Check sheet for the modelled part. Datum: model origin and axes. Units: mm. A direction names the side the tool comes from. Give positions to 0.01 mm unless a question says otherwise; leave off trailing zeros. Write each loop counter-clockwise with the first axis right and the second up, starting at its lowest first coordinate (ties: lowest second). Pieces come first, ordered by that corner, then holes. Notation, with made-up numbers: M -30.75,14.5 L -18.75,14.5 A6 cw -18.75,25.5 Z; hole C 88.5,-23.5 d7. An arc over 180 degrees is marked long. Write item = value, one per line. Start each with the question number.
1) Sectioned sample at B-B, the plane y = 0. Record the cut outline in (x, z).
2) Scan lines: L1, parallel to X at y = 0, z = -3.65; L2, parallel to Z at x = 4, y = 18; L3, parallel to Y at x = 4, z = -15. Record each from-to range of solid material in increasing order.
3) Sectioned sample at A-A, the plane z = 0. Record the cut outline in (x, y), then the cut area to 3 significant figures.
4) Sectioned sample at D-D, the plane y = -12.5. Record the cut outline in (x, z), then the cut area to 3 significant figures.
5) Draft check along Z on faces 1 (the face through (3.549, 21.728, -3.449)), 2 (the face through (-2, 2.48, -5.71)), 3 (the face through (3.45, 10.31, 16.93)). Enter one of: pulls with the +Z half, pulls with the -Z half, needs draft (parallel to the pull), parting line crosses it, or undercut.
6) Set-up check for faces 4 (the face through (3.45, 10.27, -14.17)), 5 (the face through (3.451, 19.816, -1.634)), 6 (the face through (3.451, 1.634, 19.816)): record each of +Z, -Z, +X, -X, +Y, -Y from which the full face is reachable in a straight line by a thin tool's end or side.
7) Gauge pin test, flat ends, axial feed: pin 1 (4 mm diameter, centred on x = 2.5, y = 0.5, fed in from -Z); pin 2 (2.5 mm diameter, centred on x = -2, y = 1.5, fed in from -Z); pin 3 (1.5 mm diameter, centred on y = 11.5, z = 1.5, fed in from -X). Record the tip position at first contact, or that the pin passes through.
8) Sectioned sample at C-C, the plane x = -2.5. Record the cut outline in (y, z).
from build123d import *

# Parameters (mm, degrees)
BASPROSKE_W              = 7
BASPROSKE_H              = 22
TOOTHCUT_DEPTH           = 32.890437438
TEETHCUTS_COUNT          = 20
TEETHCUTS_ANGLE          = 342
HUBNEAONESKE_R           = 7
HUBNEARONE_DEPTH         = 6.0000508
BORSKE_R                 = 3
BORE_DEPTH               = 13.0000508
CUT_EXTRUDE_3_DEPTH      = 34.466904857
CUT_EXTRUDE_3_DEPTH_BACK = 34.466904857
SKETCH_4_R               = 3.15
EXTRUDE_1_DEPTH          = 13.000051
CUT_EXTRUDE_4_DEPTH      = 32.623288929
CUT_EXTRUDE_4_DEPTH_BACK = 32.623288929
SKETCH_2_R               = 1.65
CUT_EXTRUDE_5_DEPTH      = 2


with BuildPart() as part:
    # BasProSke → Base-Revolve (revolve)
    with BuildSketch(Plane(origin=(0, 0, 0), x_dir=(1, 0, 0), z_dir=(0, 1, 0)), mode=Mode.PRIVATE) as base_revolve_sk:
        with Locations((3.5, 11)):
            Rectangle(BASPROSKE_W, BASPROSKE_H)
    revolve(base_revolve_sk.sketch.rotate(Axis((-10, 0, 0), (1, 0, 0)), 180), axis=Axis((-10, 0, 0), (1, 0, 0)))

    # TooCutSke → ToothCut (cut, through all)
    with BuildSketch(Plane(origin=(0, 0, 0), x_dir=(0, 0, -1), z_dir=(1, 0, 0))):
        with BuildLine():
            ThreePointArc((0.986171591, 17.471189616), (0, 17.499), (-0.986171591, 17.471189616))
            ThreePointArc((-0.986171591, 17.471189616), (-1.626916196, 19.798789858), (-2.932850173, 21.829260982))
            ThreePointArc((-2.932850173, 21.829260982), (0, 22.0254), (2.932850173, 21.829260982))
            ThreePointArc((2.932850173, 21.829260982), (1.626916196, 19.798789858), (0.986171591, 17.471189616))
        make_face()
    toothcut = extrude(amount=TOOTHCUT_DEPTH, mode=Mode.SUBTRACT)

    # TeethCuts: ToothCut ×20 about axis
    teethcuts_axis = Axis((-10, 0, 0), (1, 0, 0))
    for i in range(1, TEETHCUTS_COUNT):
        add(toothcut.rotate(teethcuts_axis, i * TEETHCUTS_ANGLE / (TEETHCUTS_COUNT - 1)), mode=Mode.SUBTRACT)

    # HubNeaOneSke → HubNearOne (add)
    with BuildSketch(Plane.ZY):
        with Locations(Location((0, 0, 0), (0, 0, 180))):
            Circle(HUBNEAONESKE_R)
    extrude(amount=HUBNEARONE_DEPTH)

    # BorSke → Bore (cut, symmetric)
    with BuildSketch(Plane(origin=(0, 0, 0), x_dir=(0, 0, -1), z_dir=(1, 0, 0))):
        with Locations(Location((0, 0, 0), (0, 0, 180))):
            Circle(BORSKE_R)
    extrude(amount=BORE_DEPTH, both=True, mode=Mode.SUBTRACT)

    # 草图4 → 切除-拉伸3 (cut, two sides: drawn at the far end of the back side and taken through both)
    with BuildSketch(Plane.ZY.offset(6.0000508).offset(-CUT_EXTRUDE_3_DEPTH_BACK)):
        Circle(SKETCH_4_R)
    extrude(amount=CUT_EXTRUDE_3_DEPTH + CUT_EXTRUDE_3_DEPTH_BACK, mode=Mode.SUBTRACT)

    # 草图1 → 凸台-拉伸1 (add, through all)
    with BuildSketch(Plane.ZY.offset(6.0000508)):
        with BuildLine():
            Line((2.6, 1.778341924), (2.6, -1.778341924))
            ThreePointArc((2.6, -1.778341924), (3.15, 0), (2.6, 1.778341924))
        make_face()
    extrude(amount=-EXTRUDE_1_DEPTH)

    # 草图2 → 切除-拉伸4 (cut, two sides: drawn at the far end of the back side and taken through both)
    with BuildSketch(Plane.XY.offset(-CUT_EXTRUDE_4_DEPTH_BACK)):
        with Locations((-3.5000508, 0)):
            Circle(SKETCH_2_R)
    extrude(amount=CUT_EXTRUDE_4_DEPTH + CUT_EXTRUDE_4_DEPTH_BACK, mode=Mode.SUBTRACT)

    # 草图5 → 切除-拉伸5 (cut)
    with BuildSketch(Plane.XY.offset(-7)):
        Polygon((-6.382322544, 1.704653316), (-6.417459749, -1.643793892), (-3.535188005, -3.348447209), (-0.617779056, -1.704653316), (-0.582641851, 1.643793892), (-3.464913595, 3.348447209), align=None)
    extrude(amount=CUT_EXTRUDE_5_DEPTH, mode=Mode.SUBTRACT)


solid = part.part
Data:
q1.outline = M -6,-5 L -5.15,-5 L -5.15,-3.15 L -6,-3.15 Z; M -6,2.6 L -5.15,2.6 L -5.15,7 L -6,7 Z; M -1.85,-5 L -0.6,-5 L -0.6,-7 L 0,-7 L 0,-17.5 L 7,-17.5 L 7,-3.15 L -1.85,-3.15 Z; M -1.85,2.6 L 7,2.6 L 7,17.5 L 0,17.5 L 0,7 L -1.85,7 Z
q2.L1 = -6 to -5.15, -1.85 to 7
q2.L2 = -10.47 to -7.39, -4.6 to -1.07, 1.07 to 4.6, 7.39 to 10.47
q2.L3 = -15.89 to -12.85, -9.62 to 9.62, 12.85 to 15.89
q3.outline = M -6,-7 L 0,-7 L 0,-17.5 L 7,-17.5 L 7,-3.15 L -6,-3.15 Z; M -6,3.15 L 7,3.15 L 7,17.5 L 0,17.5 L 0,7 L -6,7 Z
q3.area = 247 mm2
q4.outline = M 0,-14.78 L 7,-14.78 L 7,14.78 L 0,14.78 Z
q4.area = 207 mm2
q5.face_1 = pulls with the -Z half
q5.face_2 = needs draft
q5.face_3 = undercut
q6.face_4 = +X, -X
q6.face_5 = +X, -X, +Y
q6.face_6 = +Z, +X, -X
q7.pin_1 = -21.29
q7.pin_2 = -6.78
q7.pin_3 = 0
q8.outline = M -2.77,-6.43 L -2.77,-5 L -1.31,-5 L -1.31,-2.86 A3.15 cw -1.78,2.6 L -1.31,2.6 L -1.31,6.88 A7 ccw Z; M 1.31,-5 L 2.78,-5 L 2.78,-6.43 A7 ccw 1.31,6.88 L 1.31,2.6 L 1.78,2.6 A3.15 cw 1.31,-2.86 Z
